```python
from build123d import *

# Parameters (mm, degrees)
F0_W     = 150
F0_H     = 65
F1_DEPTH = 3
F3_W     = 5
F3_H     = 1.4
F4_DEPTH = 150.001
F2_W     = 101
F2_H     = 13
F2_H_2   = 1.7
F5_DEPTH = 0.35
F2_W_2   = 24.5
F6_DEPTH = 0.43


with BuildPart() as f1:
    # F0 (on Top) → F1 (new body)
    with BuildSketch(Plane.XY):
        Rectangle(F0_W, F0_H)
    extrude(amount=F1_DEPTH)

    # F3 (on face) → F4 (cut, through all)
    with BuildSketch(Plane.YZ.offset(75)):
        with Locations((-30, 0.7)):
            Rectangle(F3_W, F3_H)
        with Locations((30, 0.7)):
            Rectangle(F3_W, F3_H)
    extrude(amount=-F4_DEPTH, mode=Mode.SUBTRACT)

    # F2 (on face) → F5 (cut)
    with BuildSketch(Plane.XY.offset(3)):
        with Locations((12.25, 0)):
            Rectangle(F2_W, F2_H)
        with Locations((12.25, 7.35)):
            Rectangle(F2_W, F2_H_2)
    extrude(amount=-F5_DEPTH, mode=Mode.SUBTRACT)

    # F2 (on face) → F6 (cut)
    with BuildSketch(Plane.XY.offset(3)):
        with Locations((-50.5, 0)):
            Rectangle(F2_W_2, F2_H)
    extrude(amount=-F6_DEPTH, mode=Mode.SUBTRACT)


solid = f1.part
```
Could you check a few things on this model? Use its own coordinates, in mm. A direction names the side the tool comes from. Give positions to 0.01 mm unless a question says otherwise; leave off trailing zeros. Loops run counter-clockwise (first coordinate to the right, second up) from the corner with the lowest first, then second, coordinate; pieces in that order, holes last. Notation, with made-up numbers: (71, 27) - (123, 27) arc R27 cw to (123, 47) - close; hole circle Ø6 at (13, -15.5). An arc over 180 degrees is marked (long way). Use one line per item in the form item = value.
1. I want a section at B-B (x = -57). Please give me the cut outline in (y, z), and give its area (3 significant figures).
Response values:
outline = (-32.5, 1.4) - (-27.5, 1.4) - (-27.5, 0) - (27.5, 0) - (27.5, 1.4) - (32.5, 1.4) - (32.5, 3) - (6.5, 3) - (6.5, 2.57) - (-6.5, 2.57) - (-6.5, 3) - (-32.5, 3) - close
area = 175 mm²
2. I need wall thicknesses on probe 1 along Y at (x, z) = (-45.5, 0.6); probe 2 along Z at (x, y) = (-1, 4). Which ranges of each line are inside material? Lowest first, please.
Response values:
probe_1 = -27.5 to 27.5
probe_2 = 0 to 2.65
3. On a 3-axis mill with a long thin cutter (end or side, diameter ignored), from which of +Z, -Z, +X, -X, +Y, -Y can I reach the whole of each face in a straight line? I mean faces 1 (the face through (1, -30, 1.4)), 2 (the face through (-1, -7, 3)). Say none if no direction works.
Response values:
face_1 = -Z, +X, -X, -Y
face_2 = +Z, +X, -X, +Y, -Y
4. I want a section at A-A (x = 33.5). Please give me the cut outline in (y, z), and give its area (3 significant figures).
Response values:
outline = (-32.5, 1.4) - (-27.5, 1.4) - (-27.5, 0) - (27.5, 0) - (27.5, 1.4) - (32.5, 1.4) - (32.5, 3) - (8.2, 3) - (8.2, 2.65) - (-6.5, 2.65) - (-6.5, 3) - (-32.5, 3) - close
area = 176 mm²
5. I'm going to push flat-ended pins straight in: pin 1 Ø4.5 at (x, y) = (-0.5, 0) entering from +Z; pin 2 Ø4 at (x, y) = (32, -31) entering from -Z; pin 3 Ø1 at (x, z) = (3.5, 0.5) entering from +Y. Where does each tip first touch, or does it pass through?
Response values:
pin_1 = 2.65
pin_2 = 1.4
pin_3 = 27.5
6. Thinking about a two-plate mould opening in Y: for faces 3 (the face through (12, 1, 2.65)), 4 (the face through (-51, 0, 2.57)), 5 (the face through (1, 30, 1.4)), which applies, released by +Y, released by -Y, zero draft, split by the parting line, or undercut?
Response values:
face_3 = undercut
face_4 = undercut
face_5 = zero draft
